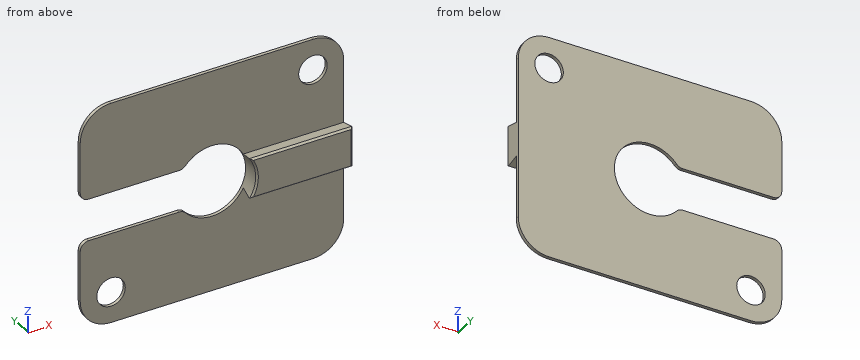
from build123d import *

# Parameters (mm, degrees)
F0_W         = 31.4
F0_H         = 26.4
F0_R         = 1.7
F1_DEPTH     = 0.4
F2_R         = 3.66
F4_DEPTH     = 25
F5_R         = 1
F7_DEPTH     = 2.2
F9_DEPTH     = 25
F10_T1_DEPTH = 13.4922434022
F10_T3_DEPTH = 5.9086731952
F10_T6_ANGLE = 83.9470182362


# Not quite as in the source:
# - a fillet or chamfer that OpenCascade refuses, or shapes differently, is made with other operations: its cross-section is extruded or revolved along the edge and cut away or added


with BuildPart() as f1:
    # F0 (on Front) → F1 (new body)
    with BuildSketch(Plane.XZ):
        Rectangle(F0_W, F0_H)
        with Locations((-12.0318713589, -9.5318713589)):
            Circle(F0_R, mode=Mode.SUBTRACT)
        with Locations((12.0318713589, 9.5318713589)):
            Circle(F0_R, mode=Mode.SUBTRACT)
    extrude(amount=F1_DEPTH)

    # F2
    f2_edges = [f1.edges().sort_by_distance(p)[0] for p in [
        (15.7, -0.2, -13.2),
        (15.7, -0.2, 13.2),
        (-15.7, -0.2, -13.2),
        (-15.7, -0.2, 13.2),
    ]]
    fillet(f2_edges, radius=F2_R)

    # F3 (on Front) → F4 (cut)
    with BuildSketch(Plane.XZ):
        with BuildLine():
            Line((-21.9406711915, -2.5), (-3.4369317712, -2.5))
            ThreePointArc((-3.4369317712, -2.5), (4.25, 0), (-3.4369317712, 2.5))
            Line((-3.4369317712, 2.5), (-21.9406711915, 2.5))
            Line((-21.9406711915, 2.5), (-21.9406711915, -2.5))
        make_face()
    extrude(amount=F4_DEPTH, mode=Mode.SUBTRACT)

    # F5
    f5_edges = [f1.edges().sort_by_distance(p)[0] for p in [
        (-3.436932, -0.2, -2.5),
        (-3.436932, -0.2, 2.5),
        (-15.7, -0.2, 2.5),
        (-15.7, -0.2, -2.5),
    ]]
    fillet(f5_edges, radius=F5_R)

    # F6 (on face) → F7 (join)
    with BuildSketch(Plane(origin=(0, 0, 0), x_dir=(-1, 0, 0), z_dir=(0, 1, 0))):
        with BuildLine():
            Line((-3.4797844761, 2.44), (-15.7, 2.44))
            Line((-15.7, 2.44), (-15.7, -2.44))
            Line((-15.7, -2.44), (-3.4797844761, -2.44))
            ThreePointArc((-3.4797844761, -2.44), (-4.25, 0), (-3.4797844761, 2.44))
        make_face()
    extrude(amount=-F7_DEPTH)

    # F8 (on face) → F9 (cut)
    with BuildSketch(Plane.YZ.offset(15.7)):
        Polygon((-0.4, 2.44), (-2.2, 2.44), (-0.4, 2.04), align=None)
        Polygon((-0.4, -2.04), (-2.2, -2.44), (-0.4, -2.44), align=None)
    extrude(amount=-F9_DEPTH, mode=Mode.SUBTRACT)

    # F10: chamfer of 0.2 on 4 edges, made by hand

    # F10_s2 → F10_t1 (cut)
    with BuildSketch(Plane.YZ.offset(2.8437705369)):
        Polygon((-1.9566139084, 2.3859142019), (-2.2, 2.1906767898), (-2.2, 2.44), align=None)
        Polygon((-2.2, -2.1906767898), (-1.9566139084, -2.3859142019), (-2.2, -2.44), align=None)
    extrude(amount=F10_T1_DEPTH, mode=Mode.SUBTRACT)

    # F10_s4 → F10_t3 (cut)
    with BuildSketch(Plane.XY.offset(-2.9543365976)):
        Polygon((15.5, -2.2), (15.7, -2), (15.7, -2.2), align=None)
    extrude(amount=F10_T3_DEPTH, mode=Mode.SUBTRACT)

    # F10_s5 → F10_t6 (revolve, cut)
    with BuildSketch(Plane(origin=(0, 0, 0), x_dir=(0, 1, 0), z_dir=(-0.6687869395, 0, -0.7434541207))):
        Polygon((-2.2, 4.45), (-2, 4.25), (-2.2, 4.25), align=None)
    revolve(axis=Axis((0, -2.2, 0), (0, -1, 0)), revolution_arc=F10_T6_ANGLE, mode=Mode.SUBTRACT)


solid = f1.part
Input: part model. Units: mm. Frame: model coordinates. Give positions to 0.01 mm unless a question says otherwise; leave off trailing zeros. Write each loop counter-clockwise with the first axis right and the second up, starting at its lowest first coordinate (ties: lowest second). Pieces come first, ordered by that corner, then holes.
Q1. Section C-C, the plane x = 6.5. Output: boundary loops of the cut face in (y, z), plus the area to 3 significant figures.
Q2. First-contact query: P1, Ø12.5, axis at x = -6, z = -6.5, coming from the -Y side; P2, Ø1, axis at y = -1.5, z = 4, coming from the -X side. Flat tips, straight axial feed; report the tip coordinate or a pass-through.
Q3. Section A-A, the plane x = 0. Output: boundary loops of the cut face in (y, z), plus the area to 3 significant figures.
Q4. Material intervals for probe 1 along Z at (x, y) = (-9, -0.1); probe 2 along Y at (x, z) = (0, -5.5); probe 3 along X at (y, z) = (-0.3, 9.75), sorted ascending.
Q5. Section B-B, the plane z = 9. Output: boundary loops of the cut face in (x, y), plus the area to 3 significant figures.
Q6. Section D-D, the plane z = 0. Output: boundary loops of the cut face in (x, y).
Filled in:
1. outline: (-2.2, -2.19) - (-1.96, -2.39) - (-0.4, -2.04) - (-0.4, -13.2) - (0, -13.2) - (0, 13.2) - (-0.4, 13.2) - (-0.4, 2.04) - (-1.96, 2.39) - (-2.2, 2.19) - close
1. area: 18.6 mm2
2. P1: stops at y = -0.4
2. P2: passes through
3. outline: (-0.4, -13.2) - (0, -13.2) - (0, -4.25) - (-0.4, -4.25) - close; (-0.4, 4.25) - (0, 4.25) - (0, 13.2) - (-0.4, 13.2) - close
3. area: 7.16 mm2
4. probe 1: z = -13.2 to -2.5, 2.5 to 13.2
4. probe 2: y = -0.4 to 0
4. probe 3: x = -15.69 to 10.35, 13.72 to 15.69
5. outline: (-15.7, -0.4) - (10.42, -0.4) - (10.42, 0) - (-15.7, 0) - close; (13.65, -0.4) - (15.7, -0.4) - (15.7, 0) - (13.65, 0) - close
5. area: 11.3 mm2
6. outline: (4.25, -2) - (4.45, -2.2) - (15.5, -2.2) - (15.7, -2) - (15.7, 0) - (4.25, 0) - close
